For this review, take the finished solid that the model builds, in its own axes (mm). A direction names the side the tool comes from. Give positions to 0.01 mm unless a question says otherwise; leave off trailing zeros. Write each loop counter-clockwise with the first axis right and the second up, starting at its lowest first coordinate (ties: lowest second). Pieces come first, ordered by that corner, then holes. Notation, with made-up numbers: M 15,-37 L 59,-37 A16 ccw 59,-20 Z; hole C 39,44 d11. An arc over 180 degrees is marked long. Write item = value, one per line.
```python
from build123d import *

# Parameters (mm, degrees)
F1_DEPTH = 63.5
F2_DEPTH = 25.4
F3_DEPTH = 7.9375
F5_R     = 6.35


with BuildPart() as f1:
    # F0 (on Front) → F1 (new body, symmetric)
    with BuildSketch(Plane.XZ):
        Polygon((-41.275, 9.525), (-41.275, -9.525), (41.275, -9.525), (41.275, 9.525), (22.225, 9.525), align=None)
    extrude(amount=F1_DEPTH, both=True)

    # F0 (on Front) → F2 (join, symmetric)
    with BuildSketch(Plane.XZ):
        with BuildLine():
            Line((22.225, 9.525), (41.275, 9.525))
            Line((41.275, 9.525), (41.275, 27.0002))
            ThreePointArc((41.275, 27.0002), (45.9246798487, 38.2255201513), (57.15, 42.8752))
            Line((57.15, 42.8752), (60.325, 42.8752))
            Line((60.325, 42.8752), (60.325, 61.9252))
            Line((60.325, 61.9252), (57.15, 61.9252))
            ThreePointArc((57.15, 61.9252), (32.4542956671, 51.6959043329), (22.225, 27.0002))
            Line((22.225, 27.0002), (22.225, 9.525))
        make_face()
        Polygon((75.878282736, 61.9252), (60.325, 61.9252), (60.325, 42.8752), (60.325, 38.1), (85.725, 38.1), (85.8768074448, 61.9252), align=None)
    extrude(amount=F2_DEPTH, both=True)

    # F0 (on Front) → F3 (join, symmetric)
    with BuildSketch(Plane.XZ):
        with BuildLine():
            add(Edge.make_bspline(
                [(-41.275, 9.525), (-40.8265404403, 41.2002727389), (25.646481663, 62.6290813088), (57.15, 61.9252)],
                knots=[0, 0, 0, 0, 111.5045361635, 111.5045361635, 111.5045361635, 111.5045361635], degree=3))
            Line((-41.275, 9.525), (22.225, 9.525))
            Line((22.225, 9.525), (22.225, 27.0002))
            ThreePointArc((22.225, 27.0002), (32.4542956671, 51.6959043329), (57.15, 61.9252))
        make_face()
    extrude(amount=F3_DEPTH, both=True)

    # F0 (on Front) → F4 (revolve)
    with BuildSketch(Plane.XZ):
        Polygon((111.125, 66.675), (85.9070718288, 66.675), (85.8768074448, 61.9252), (85.725, 38.1), (111.125, 38.1), align=None)
    revolve(axis=Axis((85.8160359144, 0, 52.3875), (0.0063715882, 0, 0.9999797012)))

    # F5
    f5_edges = [f1.edges().sort_by_distance(p)[0] for p in [
        (41.275, -63.5, 0),
        (-41.275, -63.5, 0),
        (41.275, 63.5, 0),
        (-41.275, 63.5, 0),
    ]]
    fillet(f5_edges, radius=F5_R)


solid = f1.part
```
1. Machinability: for faces 1 (the face through (22.225, 17, 18)), 2 (the face through (87.038, -0.469, 66.676)), 3 (the face through (47, -25.4, 42)), 4 (the face through (60, 4, 61.925)), which of the approach directions +Z, -Z, +X, -X, +Y, -Y give a long, thin tool a straight path to every point of the face, cutting with its end or side? Answer none if there is none.
Responses:
face_1 = +Z, -X, +Y
face_2 = +Z, +X
face_3 = +Z, +X, -X, -Y
face_4 = +Z, -X
2. Insertion check: P1, Ø6, axis at x = 82, y = 26, coming from the +Z side; P2, Ø20.5, axis at x = 71, y = -4, coming from the -Z side; P3, Ø5, axis at y = 1.5, z = 58.5, coming from the +X side (3 decimals); P4, Ø1, axis at x = 58.5, y = 8, coming from the -Z side. Each pin has a flat end and moves straight along its axis. Give the tip position at first contact, or say it passes through.
Responses:
P1 = 66.88
P2 = 38.1
P3 = 111.125
P4 = 42.88
3. For line 1 along Z through (x, y) = (62.5, -22); line 2 along Z through (x, y) = (87.5, -4.5); line 3 along X through (y, z) = (18, -0.5) (3 decimals), list the stretches that pass through material, from the lowest coordinate up. Write a range as from..to.
Responses:
line_1 = 38.1..61.93
line_2 = 38.12..66.7
line_3 = -41.275..41.275
4. We need section A-A, the plane z = 0. Write out the cut boundary in (x, y) (3 decimals), then the cut area to 3 significant figures.
Responses:
outline = M -41.275,-57.15 A6.35 ccw -34.925,-63.5 L 34.925,-63.5 A6.35 ccw 41.275,-57.15 L 41.275,57.15 A6.35 ccw 34.925,63.5 L -34.925,63.5 A6.35 ccw -41.275,57.15 Z
area = 10,400 mm2
5. We need section B-B, the plane y = -33. Write out the cut boundary in (x, z) (3 decimals), then the cut area to 3 significant figures.
Responses:
outline = M -41.275,-9.525 L 41.275,-9.525 L 41.275,9.525 L -41.275,9.525 Z
area = 1,570 mm2
